The model under review builds one solid part; all positions refer to its coordinate system, in mm. Round coordinates to 2 decimals unless told otherwise and drop trailing zeros. Loops run counter-clockwise (first coordinate to the right, second up) from the corner with the lowest first, then second, coordinate; pieces in that order, holes last. Notation, with made-up numbers: (-40, 72.5) - (-33, 72.5) arc R13 cw to (-33, 86.5) - close; hole circle Ø7 at (18, -28.5). An arc over 180 degrees is marked (long way). Answer as CSV lines item,"result".
from build123d import *

# Parameters (mm, degrees)
SKETCH_1_R      = 8
SKETCH_1_R_2    = 1.56
SKETCH_1_R_3    = 9
EXTRUDE_1_DEPTH = 3


with BuildPart() as part:
    # 草图1 → 凸台-拉伸1 (new body)
    with BuildSketch(Plane.XY):
        with BuildLine():
            Line((-27.357864376, 42), (27.357864376, 42))
            ThreePointArc((27.357864376, 42), (31.1846987, 41.238795325), (34.428932188, 39.071067812))
            Line((34.428932188, 39.071067812), (39.071067812, 34.428932188))
            ThreePointArc((39.071067812, 34.428932188), (41.238795325, 31.1846987), (42, 27.357864376))
            Line((42, 27.357864376), (42, 24.357864376))
            ThreePointArc((42, 24.357864376), (42.878679656, 22.236544033), (45, 21.357864376))
            Line((45, 21.357864376), (74, 21.357864376))
            ThreePointArc((74, 21.357864376), (76.121320344, 20.47918472), (77, 18.357864376))
            Line((77, 18.357864376), (77, -18.357864376))
            ThreePointArc((77, -18.357864376), (76.121320344, -20.47918472), (74, -21.357864376))
            Line((74, -21.357864376), (45, -21.357864376))
            ThreePointArc((45, -21.357864376), (42.878679656, -22.236544033), (42, -24.357864376))
            Line((42, -24.357864376), (42, -27.357864376))
            ThreePointArc((42, -27.357864376), (41.238795325, -31.1846987), (39.071067812, -34.428932188))
            Line((39.071067812, -34.428932188), (34.428932188, -39.071067812))
            ThreePointArc((34.428932188, -39.071067812), (31.1846987, -41.238795325), (27.357864376, -42))
            Line((27.357864376, -42), (-27.357864376, -42))
            ThreePointArc((-27.357864376, -42), (-31.1846987, -41.238795325), (-34.428932188, -39.071067812))
            Line((-34.428932188, -39.071067812), (-39.071067812, -34.428932188))
            ThreePointArc((-39.071067812, -34.428932188), (-41.238795325, -31.1846987), (-42, -27.357864376))
            Line((-42, -27.357864376), (-42, -24.357864376))
            ThreePointArc((-42, -24.357864376), (-42.878679656, -22.236544033), (-45, -21.357864376))
            Line((-45, -21.357864376), (-74, -21.357864376))
            ThreePointArc((-74, -21.357864376), (-76.121320344, -20.47918472), (-77, -18.357864376))
            Line((-77, -18.357864376), (-77, 18.357864376))
            ThreePointArc((-77, 18.357864376), (-76.121320344, 20.47918472), (-74, 21.357864376))
            Line((-74, 21.357864376), (-45, 21.357864376))
            ThreePointArc((-45, 21.357864376), (-42.878679656, 22.236544033), (-42, 24.357864376))
            Line((-42, 24.357864376), (-42, 27.357864376))
            ThreePointArc((-42, 27.357864376), (-41.238795325, 31.1846987), (-39.071067812, 34.428932188))
            Line((-39.071067812, 34.428932188), (-34.428932188, 39.071067812))
            ThreePointArc((-34.428932188, 39.071067812), (-31.1846987, 41.238795325), (-27.357864376, 42))
        make_face()
        Circle(SKETCH_1_R, mode=Mode.SUBTRACT)
        with Locations((-26.196699141, 36.803300859)):
            Circle(SKETCH_1_R_2, mode=Mode.SUBTRACT)
        with Locations((-36.803300859, 26.196699141)):
            Circle(SKETCH_1_R_2, mode=Mode.SUBTRACT)
        with Locations(Location((26.196699141, 36.803300859, 0), (0, 0, 180))):
            Circle(SKETCH_1_R_2, mode=Mode.SUBTRACT)
        with Locations(Location((36.803300859, 26.196699141, 0), (0, 0, 180))):
            Circle(SKETCH_1_R_2, mode=Mode.SUBTRACT)
        with Locations((36.803300859, -26.196699141)):
            Circle(SKETCH_1_R_2, mode=Mode.SUBTRACT)
        with Locations((26.196699141, -36.803300859)):
            Circle(SKETCH_1_R_2, mode=Mode.SUBTRACT)
        with Locations(Location((-26.196699141, -36.803300859, 0), (0, 0, 180))):
            Circle(SKETCH_1_R_2, mode=Mode.SUBTRACT)
        with Locations(Location((-36.803300859, -26.196699141, 0), (0, 0, 180))):
            Circle(SKETCH_1_R_2, mode=Mode.SUBTRACT)
        with Locations((0, 36.803300859)):
            Circle(SKETCH_1_R_2, mode=Mode.SUBTRACT)
        with Locations(Location((36.803300859, 0, 0), (0, 0, 180))):
            Circle(SKETCH_1_R_2, mode=Mode.SUBTRACT)
        with Locations(Location((0, -36.803300859, 0), (0, 0, 180))):
            Circle(SKETCH_1_R_2, mode=Mode.SUBTRACT)
        with Locations((-36.803300859, 0)):
            Circle(SKETCH_1_R_2, mode=Mode.SUBTRACT)
        with Locations((-60, 0)):
            Circle(SKETCH_1_R_3, mode=Mode.SUBTRACT)
        with Locations((60, 0)):
            Circle(SKETCH_1_R_3, mode=Mode.SUBTRACT)
        with BuildLine():
            Line((-17.5, 24.05), (17.5, 24.05))
            ThreePointArc((17.5, 24.05), (19.05, 22.5), (17.5, 20.95))
            Line((17.5, 20.95), (-17.5, 20.95))
            ThreePointArc((-17.5, 20.95), (-19.05, 22.5), (-17.5, 24.05))
        make_face(mode=Mode.SUBTRACT)
        with BuildLine():
            Line((-17.5, -24.05), (17.5, -24.05))
            ThreePointArc((17.5, -24.05), (19.05, -22.5), (17.5, -20.95))
            Line((17.5, -20.95), (-17.5, -20.95))
            ThreePointArc((-17.5, -20.95), (-19.05, -22.5), (-17.5, -24.05))
        make_face(mode=Mode.SUBTRACT)
        with BuildLine():
            Line((24.05, -17.5), (24.05, 17.5))
            ThreePointArc((24.05, 17.5), (22.5, 19.05), (20.95, 17.5))
            Line((20.95, 17.5), (20.95, -17.5))
            ThreePointArc((20.95, -17.5), (22.5, -19.05), (24.05, -17.5))
        make_face(mode=Mode.SUBTRACT)
        with BuildLine():
            Line((-24.05, -17.5), (-24.05, 17.5))
            ThreePointArc((-24.05, 17.5), (-22.5, 19.05), (-20.95, 17.5))
            Line((-20.95, 17.5), (-20.95, -17.5))
            ThreePointArc((-20.95, -17.5), (-22.5, -19.05), (-24.05, -17.5))
        make_face(mode=Mode.SUBTRACT)
        with BuildLine():
            Line((8.903984489, 11.096015511), (13.903984489, 16.096015511))
            ThreePointArc((13.903984489, 16.096015511), (16.096015511, 16.096015511), (16.096015511, 13.903984489))
            Line((16.096015511, 13.903984489), (11.096015511, 8.903984489))
            ThreePointArc((11.096015511, 8.903984489), (8.903984489, 8.903984489), (8.903984489, 11.096015511))
        make_face(mode=Mode.SUBTRACT)
        with BuildLine():
            Line((-8.903984489, 11.096015511), (-13.903984489, 16.096015511))
            ThreePointArc((-13.903984489, 16.096015511), (-16.096015511, 16.096015511), (-16.096015511, 13.903984489))
            Line((-16.096015511, 13.903984489), (-11.096015511, 8.903984489))
            ThreePointArc((-11.096015511, 8.903984489), (-8.903984489, 8.903984489), (-8.903984489, 11.096015511))
        make_face(mode=Mode.SUBTRACT)
        with BuildLine():
            Line((-8.903984489, -11.096015511), (-13.903984489, -16.096015511))
            ThreePointArc((-13.903984489, -16.096015511), (-16.096015511, -16.096015511), (-16.096015511, -13.903984489))
            Line((-16.096015511, -13.903984489), (-11.096015511, -8.903984489))
            ThreePointArc((-11.096015511, -8.903984489), (-8.903984489, -8.903984489), (-8.903984489, -11.096015511))
        make_face(mode=Mode.SUBTRACT)
        with BuildLine():
            Line((8.903984489, -11.096015511), (13.903984489, -16.096015511))
            ThreePointArc((13.903984489, -16.096015511), (16.096015511, -16.096015511), (16.096015511, -13.903984489))
            Line((16.096015511, -13.903984489), (11.096015511, -8.903984489))
            ThreePointArc((11.096015511, -8.903984489), (8.903984489, -8.903984489), (8.903984489, -11.096015511))
        make_face(mode=Mode.SUBTRACT)
        with BuildLine():
            Line((-33.211093213, 22.604491495), (-22.604491495, 33.211093213))
            ThreePointArc((-22.604491495, 33.211093213), (-19.18230507, 33.211093213), (-19.18230507, 29.788906787))
            Line((-19.18230507, 29.788906787), (-29.788906787, 19.18230507))
            ThreePointArc((-29.788906787, 19.18230507), (-33.211093213, 19.18230507), (-33.211093213, 22.604491495))
        make_face(mode=Mode.SUBTRACT)
        with BuildLine():
            Line((33.211093213, 22.604491495), (22.604491495, 33.211093213))
            ThreePointArc((22.604491495, 33.211093213), (19.18230507, 33.211093213), (19.18230507, 29.788906787))
            Line((19.18230507, 29.788906787), (29.788906787, 19.18230507))
            ThreePointArc((29.788906787, 19.18230507), (33.211093213, 19.18230507), (33.211093213, 22.604491495))
        make_face(mode=Mode.SUBTRACT)
        with BuildLine():
            Line((-33.211093213, -22.604491495), (-22.604491495, -33.211093213))
            ThreePointArc((-22.604491495, -33.211093213), (-19.18230507, -33.211093213), (-19.18230507, -29.788906787))
            Line((-19.18230507, -29.788906787), (-29.788906787, -19.18230507))
            ThreePointArc((-29.788906787, -19.18230507), (-33.211093213, -19.18230507), (-33.211093213, -22.604491495))
        make_face(mode=Mode.SUBTRACT)
        with BuildLine():
            Line((33.211093213, -22.604491495), (22.604491495, -33.211093213))
            ThreePointArc((22.604491495, -33.211093213), (19.18230507, -33.211093213), (19.18230507, -29.788906787))
            Line((19.18230507, -29.788906787), (29.788906787, -19.18230507))
            ThreePointArc((29.788906787, -19.18230507), (33.211093213, -19.18230507), (33.211093213, -22.604491495))
        make_face(mode=Mode.SUBTRACT)
    extrude(amount=EXTRUDE_1_DEPTH)


solid = part.part
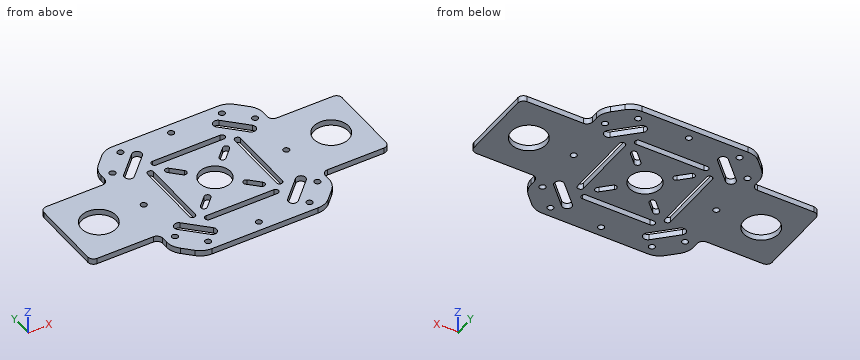
1. Take a section at D-D (z = 1.5). State how many separate pieces and enclosed holes the cut face has, plus the area to 3 significant figures.
Numbers:
separate pieces,"1"
enclosed holes,"27"
area,"8,060 mm²"
2. Take a section at C-C (y = -31.5). State the section outline as (x, z) points, plus the area to 3 significant figures.
Numbers:
outline,"(-41.1, 0) - (-24.32, 0) - (-24.32, 3) - (-41.1, 3) - close; (-18.47, 0) - (18.47, 0) - (18.47, 3) - (-18.47, 3) - close; (24.32, 0) - (41.1, 0) - (41.1, 3) - (24.32, 3) - close"
area,"212 mm²"
3. Clearance check with flat-ended pins moving along their axes: pin 1 (2.5 mm diameter, centred on x = 36.8, y = 26.2, fed in from -Z); pin 2 (1.5 mm diameter, centred on y = -26.5, z = 1.5, fed in from +X); pin 3 (1.5 mm diameter, centred on x = 64, z = 1.5, fed in from +Y); pin 4 (0.9 mm diameter, centred on y = -25.5, z = 1, fed in from -X). State where each tip first meets the part, or that it passes through.
Numbers:
pin 1,"passes through"
pin 2,"stops at x = 42"
pin 3,"stops at y = 21.36"
pin 4,"stops at x = -42"
4. Take a section at A-A (x = 0). State the section outline as (y, z) points.
Numbers:
outline,"(-42, 0) - (-38.36, 0) - (-38.36, 3) - (-42, 3) - close; (-35.24, 0) - (-24.05, 0) - (-24.05, 3) - (-35.24, 3) - close; (-20.95, 0) - (-8, 0) - (-8, 3) - (-20.95, 3) - close; (8, 0) - (20.95, 0) - (20.95, 3) - (8, 3) - close; (24.05, 0) - (35.24, 0) - (35.24, 3) - (24.05, 3) - close; (38.36, 0) - (42, 0) - (42, 3) - (38.36, 3) - close"
5. Take a section at B-B (x = -61). State the section outline as (y, z) points, plus the area to 3 significant figures.
Numbers:
outline,"(-21.36, 0) - (-8.94, 0) - (-8.94, 3) - (-21.36, 3) - close; (8.94, 0) - (21.36, 0) - (21.36, 3) - (8.94, 3) - close"
area,"74.5 mm²"
6. Wall thickness on probe 1 along Y at (x, z) = (0, 1.55); probe 2 along Y at (x, z) = (-60, 0.6); probe 3 along Y at (x, z) = (26, 2.4): over which ranges is each line inside the solid? List them lowest first.
Numbers:
probe 1,"y = -42 to -38.36, -35.24 to -24.05, -20.95 to -8, 8 to 20.95, 24.05 to 35.24, 38.36 to 42"
probe 2,"y = -21.36 to -9, 9 to 21.36"
probe 3,"y = -42 to -38.35, -35.26 to -29.82, -22.97 to 22.97, 29.82 to 35.26, 38.35 to 42"
